Design review of the part built by this model. Coordinates are the model's own, in mm. A direction names the side the tool comes from. Give positions to 0.01 mm unless a question says otherwise; leave off trailing zeros. Loops run counter-clockwise (first coordinate to the right, second up) from the corner with the lowest first, then second, coordinate; pieces in that order, holes last. Notation, with made-up numbers: (35, 88) -> (73, 88) arc R16 ccw to (73, 93) -> close; hole circle Ø5 at (55.5, 80). An arc over 180 degrees is marked (long way). Answer as CSV lines item,"result".
from build123d import *

# Parameters (mm, degrees)
BOSS_EXTRUDE1_DEPTH    = 38.1
CONVERT_SOLID1_DEPTH   = 38.1
CONVERT_SOLID1_2_DEPTH = 38.1


# Read off the part's stored shape, not the designer's step: Convert-Solid1
with BuildPart() as part:
    # Sketch1 → Boss-Extrude1 (new body)
    with BuildSketch(Plane(origin=(0, 0, 0), x_dir=(0, 0, -1), z_dir=(1, 0, 0))):
        Polygon((-1.524, 38.1), (-1.524, 1.524), (-38.1, 1.524), (-38.1, 0), (0, 0), (0, 38.1), align=None)
    extrude(amount=BOSS_EXTRUDE1_DEPTH)

    # Convert-Solid1 outline → Convert-Solid1 (cut)
    with BuildSketch(Plane.YZ):
        with BuildLine():
            ThreePointArc((3.048, 0), (0.892738531, 0.892738531), (0, 3.048))
            Line((0, 3.048), (0, 0))
            Line((0, 0), (3.048, 0))
        make_face()
    extrude(amount=CONVERT_SOLID1_DEPTH, mode=Mode.SUBTRACT)

    # Convert-Solid1 2 outline → Convert-Solid1 2 (add)
    with BuildSketch(Plane.YZ):
        with BuildLine():
            ThreePointArc((3.048, 1.524), (1.970369265, 1.970369265), (1.524, 3.048))
            Line((1.524, 3.048), (1.524, 1.524))
            Line((1.524, 1.524), (3.048, 1.524))
        make_face()
    extrude(amount=CONVERT_SOLID1_2_DEPTH)


solid = part.part
Q1. We need section A-A, the plane x = 11. State the section outline as (y, z) points.
Filled sheet:
outline,"(0, 3.05) arc R3.05 ccw to (3.05, 0) -> (38.1, 0) -> (38.1, 1.52) -> (3.05, 1.52) arc R1.52 cw to (1.52, 3.05) -> (1.52, 38.1) -> (0, 38.1) -> close"
Q2. Clearance check with a flat-ended pin moving along its axis: pin 1 Ø1 at (x, z) = (23.5, 16.5) entering from +Y. State where the tip first meets the part, or that it passes through.
Filled sheet:
pin 1,"stops at y = 1.52"
Q3. To check wall thickness, follow probe 1 along Z at (x, y) = (8, 33); probe 2 along Z at (x, y) = (29, 2.5). State the ranges of each line that lie inside material, in increasing order. Write a range as from..to.
Filled sheet:
probe 1,"z = 0..1.52"
probe 2,"z = 0.05..1.63"
Q4. We need section B-B, the plane z = 15.5. State the section outline as (x, y) points, and give its area (3 significant figures).
Filled sheet:
outline,"(0, 0) -> (38.1, 0) -> (38.1, 1.52) -> (0, 1.52) -> close"
area,"58.1 mm^2"
Q5. For faces 1 (the flat face through (19, 21, 1.524)), 2 (the cylindrical face through (18.783, 0.917, 0.869)), list the 3-axis set-ups (+Z, -Z, +X, -X, +Y, -Y) from which the entire face can be reached by the end or side of a thin tool; tool diameter is ignored.
Filled sheet:
face 1,"+Z, +X, -X, +Y"
face 2,"-Z, +X, -X, -Y"
